```python
from build123d import *

# Parameters (mm, degrees)
BOSS_EXTRUDE1_DEPTH      = 50.8
BOSS_EXTRUDE1_DEPTH_BACK = 6.35
SKETCH1_W                = 61.468
SKETCH1_H                = 61.468
SKETCH1_3_W              = 41.656
SKETCH1_3_H              = 41.656
CUT_EXTRUDE1_DEPTH       = 67.856544272
SKETCH5_W                = 38.1
SKETCH5_H                = 38.1
CUT_EXTRUDE3_DEPTH       = 72.800278635
SKETCH7_W                = 51.308
SKETCH7_H                = 51.308
CUT_EXTRUDE4_DEPTH       = 55.111902709


with BuildPart() as part:
    # Sketch1 → Boss-Extrude1 (new, two sides: drawn at the far end of the back side and taken through both)
    with BuildSketch(Plane.XY.offset(-BOSS_EXTRUDE1_DEPTH_BACK)):
        Rectangle(SKETCH1_W, SKETCH1_H)
    extrude(amount=BOSS_EXTRUDE1_DEPTH + BOSS_EXTRUDE1_DEPTH_BACK)

    # Sketch1<3> → Cut-Extrude1 (cut, through all)
    with BuildSketch(Plane.XY):
        Rectangle(SKETCH1_3_W, SKETCH1_3_H)
    extrude(amount=CUT_EXTRUDE1_DEPTH, mode=Mode.SUBTRACT)

    # Sketch5 → Cut-Extrude3 (cut, through all)
    with BuildSketch(Plane(origin=(0, 0, -6.35), x_dir=(-1, 0, 0), z_dir=(0, 0, -1))):
        Rectangle(SKETCH5_W, SKETCH5_H)
    extrude(amount=-CUT_EXTRUDE3_DEPTH, mode=Mode.SUBTRACT)

    # Sketch7 → Cut-Extrude4 (cut, through all)
    with BuildSketch(Plane(origin=(0, 0, 18.5674), x_dir=(-1, 0, 0), z_dir=(0, 0, -1))):
        Rectangle(SKETCH7_W, SKETCH7_H)
    extrude(amount=-CUT_EXTRUDE4_DEPTH, mode=Mode.SUBTRACT)


solid = part.part
```
Check sheet for the modelled part. Datum: model origin and axes. Units: mm. A direction names the side the tool comes from. Coordinates: 2 decimals unless noted, no trailing zeros. Order: outer loops, then holes, each group sorted by start corner. A loop starts at its lowest first (then second) coordinate and runs counter-clockwise, first axis right, second up. Notation, with made-up numbers: (52.25, -38.75) -> (108.25, -38.75) arc R9 cw to (108.25, -25.75) -> close; hole circle Ø8 at (-0.5, 83.25). An arc over 180 degrees is marked (long way). Write item = value, one per line. Start each with the question number.
1) Material ranges on L1, parallel to X at y = 2.5, z = 21; L2, parallel to Y at x = 14.5, z = -0.5, recorded low to high.
2) Cross-section at A-A (x = -7). Enter the section's corners in (y, z), then the cut area to 3 significant figures.
3) Cross-section at D-D (y = 22). Enter the section's corners in (x, z).
4) Access from +Z, -Z, +X, -X, +Y, -Y to the whole of each face (thin tool, end or side, straight path). Record for faces 1 (the flat face through (0, -25.654, 34)), 2 (the flat face through (0, 19.05, -3)), 3 (the flat face through (30.734, 0, 22)).
5) Cross-section at C-C (z = 6.5). Enter the section's corners in (x, y), then the cut area to 3 significant figures.
6) Mould release check, pull along Y, two halves, no side actions. Record for faces 4 (the flat face through (-30.734, 0, 22)), 5 (the flat face through (19.05, 0, -3)), 6 (the flat face through (0, 30.734, 22)): +Y half, -Y half, draft (parallel to the pull), parting line (faces both ways), or undercut.
7) Go/stop test with a flat-tipped pin: P1, Ø4, axis at x = 21, y = 12, coming from the +Z side. Record where the tip stops, or that it passes through.
Ans:
q1.L1 = -30.73 to -25.65, 25.65 to 30.73
q1.L2 = -30.73 to -19.05, 19.05 to 30.73
q2.outline = (-30.73, -6.35) -> (-19.05, -6.35) -> (-19.05, 0) -> (-20.83, 0) -> (-20.83, 18.57) -> (-25.65, 18.57) -> (-25.65, 50.8) -> (-30.73, 50.8) -> close; (19.05, -6.35) -> (30.73, -6.35) -> (30.73, 50.8) -> (25.65, 50.8) -> (25.65, 18.57) -> (20.83, 18.57) -> (20.83, 0) -> (19.05, 0) -> close
q2.area = 844 mm²
q3.outline = (-30.73, -6.35) -> (30.73, -6.35) -> (30.73, 50.8) -> (25.65, 50.8) -> (25.65, 18.57) -> (-25.65, 18.57) -> (-25.65, 50.8) -> (-30.73, 50.8) -> close
q4.face_1 = +Z
q4.face_2 = +Z, -Z
q4.face_3 = +Z, -Z, +X, +Y, -Y
q5.outline = (-30.73, -30.73) -> (30.73, -30.73) -> (30.73, 30.73) -> (-30.73, 30.73) -> close; hole (-20.83, -20.83) -> (20.83, -20.83) -> (20.83, 20.83) -> (-20.83, 20.83) -> close
q5.area = 2,040 mm²
q6.face_4 = draft
q6.face_5 = undercut
q6.face_6 = +Y half
q7.P1 = 18.57
